Can you work these out from the drawing? Everything is in mm from the part's minimum corner. Give positions to 0.01 mm unless a question says otherwise; leave off trailing zeros. Write each loop counter-clockwise with the first axis right and the second up, starting at its lowest first coordinate (ties: lowest second). Pieces come first, ordered by that corner, then holes. Notation, with made-up numbers: (61, -10.5) -> (98, -10.5) arc R10 ccw to (98, 7.5) -> close; hole circle Ø3 at (73.5, 17). An arc over 180 degrees is marked (long way). Return JSON: item names as keys, results as strings.
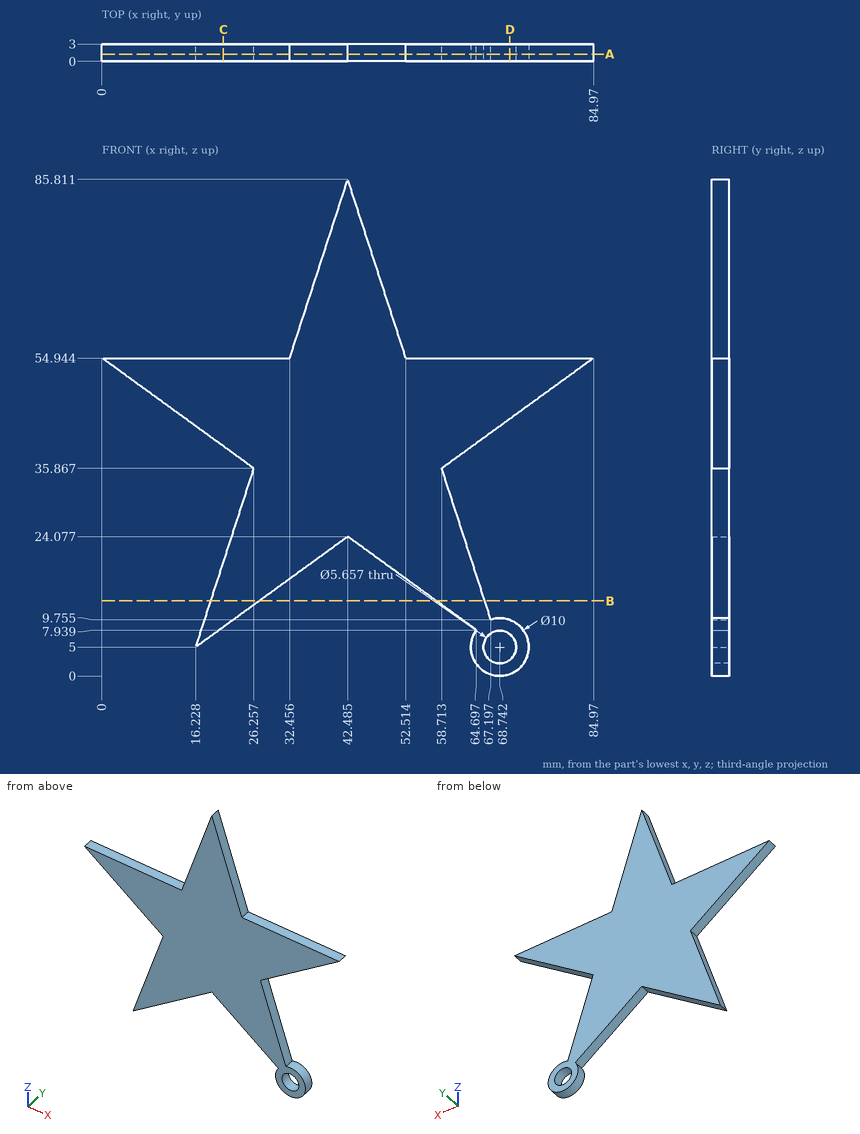
1. Suppose I cut it at D-D, the plane x = 70.5. List the corners of the cut face in (y, z) for me (1 decimal).
Taken from the geometry:
{"outline": "(0, 0.3) -> (3, 0.3) -> (3, 2.8) -> (0, 2.8) -> close; (0, 7.2) -> (3, 7.2) -> (3, 9.7) -> (0, 9.7) -> close; (0, 44.4) -> (3, 44.4) -> (3, 54.9) -> (0, 54.9) -> close"}
2. If I drill on line 1 (Z direction, x = 71, y = 2.65) (1 decimal); line 2 (Z direction, x = 76.5, y = 0.15) (1 decimal); line 3 (X direction, y = 1.1, z = 67), over which ranges is the centre line in solid material (lowest first)? Write a range as [from, to].
Taken from the geometry:
{"line 1": "z = [0.5, 3.3], [6.7, 9.5], [44.8, 54.9]", "line 2": "z = [48.8, 54.9]", "line 3": "x = [36.37, 48.6]"}
3. Suppose I cut it at B-B, the plane z = 13. List the corners of the cut face in (x, y) for me.
Taken from the geometry:
{"outline": "(18.83, 0) -> (27.24, 0) -> (27.24, 3) -> (18.83, 3) -> close; (57.73, 0) -> (66.14, 0) -> (66.14, 3) -> (57.73, 3) -> close"}
4. Suppose I cut it at A-A, the plane y = 1.25. List the corners of the cut face in (x, z) for me (1 decimal).
Taken from the geometry:
{"outline": "(0, 54.9) -> (26.3, 35.9) -> (16.2, 5) -> (42.5, 24.1) -> (64.7, 7.9) arc R5 ccw (long way) to (67.2, 9.8) -> (58.7, 35.9) -> (85, 54.9) -> (52.5, 54.9) -> (42.5, 85.8) -> (32.5, 54.9) -> close; hole circle Ø5.7 at (68.7, 5)"}
5. For pin 1 Ø1.5 at (y, z) = (2, 49.5) entering from +X; pin 2 Ø5 at (x, z) = (68.74, 5) entering from +Y; pin 3 Ø0.9 at (x, y) = (66.5, 1) entering from +Z, each with a flat end and sliding along its axis, tell me the tip position at first contact or that it passes through.
Taken from the geometry:
{"pin 1": "stops at x = 78.51", "pin 2": "passes through", "pin 3": "stops at z = 54.94"}
6. Suppose I cut it at C-C, the plane x = 21. List the corners of the cut face in (y, z) for me (1 decimal).
Taken from the geometry:
{"outline": "(0, 8.5) -> (3, 8.5) -> (3, 19.7) -> (0, 19.7) -> close; (0, 39.7) -> (3, 39.7) -> (3, 54.9) -> (0, 54.9) -> close"}
